Build history of the part. All positions in model axes, mm. A direction names the side the tool comes from. Give positions to 0.01 mm unless a question says otherwise; leave off trailing zeros. Loops run counter-clockwise (first coordinate to the right, second up) from the corner with the lowest first, then second, coordinate; pieces in that order, holes last. Notation, with made-up numbers: M 10.5,81.25 L 22.5,81.25 A10 ccw 22.5,96.25 Z; hole C 29.25,81.25 d9. An arc over 180 degrees is marked long. Answer as a JSON object with one key per item and string values. Group by question number.
1. Slice it at A-A (y = 17). List the corners of the cut face in (x, z), then the cut area to 3 significant figures.
2. Slice it at C-C (z = 17). List the corners of the cut face in (x, y).
3. Drill centre lines: line 1 along Y through (x, z) = (0, 9.25); line 2 along X through (y, z) = (-7, -14.5); line 3 along X through (y, z) = (-30, 13.5). Where is each one in solid material? Low to high. Write a range as [from, to].
4. 3-axis set-ups, long thin cutter, end or side, ignore diameter. For faces 1 (the face through (0.9, -26, 12.4)), 2 (the face through (-8, 0, 0)), 3 (the face through (-15, 1, 15)): which of +Z, -Z, +X, -X, +Y, -Y reach the whole face in a straight line?
5. Drop flat-ended pins along their axis: pin 1 Ø2.5 at (x, y) = (0.5, 30.5) entering from +Z; pin 2 Ø22 at (x, y) = (-25, -5.5) entering from +Z; pin 3 Ø9 at (x, y) = (-25.5, -10) entering from +Z; pin 4 Ø10 at (y, z) = (-8.5, -7) entering from -X. Give the stop position or say it passes through.
6. Slice it at B-B (x = -29.5). List the corners of the cut face in (y, z), then the cut area to 3 significant figures.
7. Mould opens along X. For faces 4 (the face through (14.765, -34.921, 0.315)), 5 (the face through (-6, -18, 0)), 6 (the face through (-15, 1, -8)) say: released by +X, released by -X, zero draft, split by the parting line, or undercut.
8. Slice it at D-D (y = -25). List the corners of the cut face in (x, z), then the cut area to 3 significant figures.
from build123d import *

# Parameters (mm, degrees)
CROQUIS1_R              = 4.1
SALIENTE_EXTRUIR1_DEPTH = 22.5
CROQUIS2_W              = 20
CROQUIS2_H              = 4
SALIENTE_EXTRUIR2_DEPTH = 80
REDONDEO1_R             = 2
CROQUIS3_R              = 4.1
SALIENTE_EXTRUIR3_DEPTH = 25


with BuildPart() as part:
    # Croquis1 → Saliente-Extruir1 (new, symmetric)
    with BuildSketch(Plane.XY):
        with BuildLine():
            Line((14.121320343, 35.878679656), (10.878679656, 39.121320344))
            ThreePointArc((10.878679656, 39.121320344), (9.90540961, 39.771638598), (8.757359313, 40))
            Line((8.757359313, 40), (-15, 40))
            Line((-15, 40), (-15, -40))
            Line((-15, -40), (8.757359313, -40))
            ThreePointArc((8.757359313, -40), (9.90540961, -39.771638598), (10.878679656, -39.121320344))
            Line((10.878679656, -39.121320344), (14.121320343, -35.878679656))
            ThreePointArc((14.121320343, -35.878679656), (14.771638597, -34.90540961), (15, -33.757359313))
            Line((15, -33.757359313), (15, 33.757359313))
            ThreePointArc((15, 33.757359313), (14.771638597, 34.90540961), (14.121320343, 35.878679656))
        make_face()
        with Locations(Location((0, 30, 0), (0, 0, 180))):
            Circle(CROQUIS1_R, mode=Mode.SUBTRACT)
        with Locations(Location((0, -30, 0), (0, 0, 180))):
            Circle(CROQUIS1_R, mode=Mode.SUBTRACT)
        Polygon((-4, -20), (-8, -16), (-8, 16), (-4, 20), (4, 20), (8, 16), (8, -16), (4, -20), align=None, mode=Mode.SUBTRACT)
    extrude(amount=SALIENTE_EXTRUIR1_DEPTH, both=True)

    # Croquis2 → Saliente-Extruir2 (add)
    with BuildSketch(Plane(origin=(0, 40, 0), x_dir=(1, 0, 0), z_dir=(0, 1, 0))):
        with Locations((-25, 20.5)):
            Rectangle(CROQUIS2_W, CROQUIS2_H)
        with Locations((-25, -3.5)):
            Rectangle(CROQUIS2_W, CROQUIS2_H)
    extrude(amount=-SALIENTE_EXTRUIR2_DEPTH)

    # Redondeo1
    redondeo1_edges = [part.edges().sort_by_distance(p)[0] for p in [
        (-15, 0, 5.5),
    ]]
    fillet(redondeo1_edges, radius=REDONDEO1_R)

    # Croquis3 → Saliente-Extruir3 (add)
    with BuildSketch(Plane(origin=(0, 0, -22.5), x_dir=(-1, 0, 0), z_dir=(0, 0, -1))):
        with Locations((0, -30)):
            Circle(CROQUIS3_R)
        with Locations((0, 30)):
            Circle(CROQUIS3_R)
    extrude(amount=-SALIENTE_EXTRUIR3_DEPTH)


solid = part.part
Established:
{
 "1": {"outline": "M -35,-22.5 L -7,-22.5 L -7,22.5 L -15,22.5 L -15,7.5 A2 cw -17,5.5 L -35,5.5 L -35,1.5 L -15,1.5 L -15,-18.5 L -35,-18.5 Z; M 7,-22.5 L 15,-22.5 L 15,22.5 L 7,22.5 Z", "area": "881 mm^2"},
 "2": {"outline": "M -15,-40 L 8.76,-40 A3 ccw 10.88,-39.12 L 14.12,-35.88 A3 ccw 15,-33.76 L 15,33.76 A3 ccw 14.12,35.88 L 10.88,39.12 A3 ccw 8.76,40 L -15,40 Z; hole M -8,-16 L -4,-20 L 4,-20 L 8,-16 L 8,16 L 4,20 L -4,20 L -8,16 Z; hole C 0,-30 d8.2; hole C 0,30 d8.2"},
 "3": {"line 1": "y = [-40, -34.1], [-25.9, -20], [20, 25.9], [34.1, 40]", "line 2": "x = [-15, -8], [8, 15]", "line 3": "x = [-15, -4.1], [4.1, 15]"},
 "4": {"face 1": "+Z", "face 2": "+Z, -Z", "face 3": "+Z, -X, +Y, -Y"},
 "5": {"pin 1": "stops at z = 2.5", "pin 2": "stops at z = 22.5", "pin 3": "stops at z = 5.5", "pin 4": "stops at x = -15"},
 "6": {"outline": "M -40,-22.5 L 40,-22.5 L 40,-18.5 L -40,-18.5 Z; M -40,1.5 L 40,1.5 L 40,5.5 L -40,5.5 Z", "area": "640 mm^2"},
 "7": {"face 4": "released by +X", "face 5": "undercut", "face 6": "released by -X"},
 "8": {"outline": "M -35,-22.5 L 15,-22.5 L 15,22.5 L -15,22.5 L -15,7.5 A2 cw -17,5.5 L -35,5.5 L -35,1.5 L -15,1.5 L -15,-18.5 L -35,-18.5 Z", "area": "1,510 mm^2"}
}
